```python
from build123d import *

# Parameters (mm, degrees)
F9_DEPTH = 60


with BuildPart() as f3:
    # F0 (on Top) → F3 section 0
    with BuildSketch(Plane.XY):
        Polygon((75, 43.3012701892), (0, 86.6025403784), (-75, 43.3012701892), (-75, -43.3012701892), (0, -86.6025403784), (75, -43.3012701892), align=None)
    # F2 (on offset) → F3 section 1
    with BuildSketch(Plane.XY.offset(50)):
        Polygon((40.3265245185, 23.2825297862), (0, 46.5650595725), (-40.3265245185, 23.2825297862), (-40.3265245185, -23.2825297862), (0, -46.5650595725), (40.3265245185, -23.2825297862), align=None)
    loft()

    # F3_face (on face) → F6 section 0
    with BuildSketch(Plane.XY.offset(50), mode=Mode.PRIVATE) as f6_s0:
        Polygon((40.3265245185, -23.2825297862), (40.3265245185, 23.2825297862), (0, 46.5650595725), (-40.3265245185, 23.2825297862), (-40.3265245185, -23.2825297862), (0, -46.5650595725), align=None)
    loft([f6_s0.sketch, Vertex(-50.6460405886, 55.1455877721, 115)])

    # F8 (on offset) → F9 (join)
    with BuildSketch(Plane(origin=(15.7716130811, -27.3172351738, 55.0342066068), x_dir=(0.9685974066, 0.1105451644, -0.2227079489), z_dir=(0.2486343981, -0.4306474099, 0.8675965332))):
        Polygon((25.1611340791, 2.2766380571), (-68.6507374048, 100.4471331835), (-16.3836460561, -19.314782694), align=None)
    extrude(amount=F9_DEPTH)


solid = f3.part
```
Geometry: final body of the model. Coordinates: model frame, mm. A direction names the side the tool comes from. Coordinates: 2 decimals unless noted, no trailing zeros. Order: outer loops, then holes, each group sorted by start corner. A loop starts at its lowest first (then second) coordinate and runs counter-clockwise, first axis right, second up. Notation, with made-up numbers: (-7, 52) -> (47, 52) arc R25 cw to (47, 84) -> close; hole circle Ø6 at (61, 22). An arc over 180 degrees is marked (long way). Answer in a Markdown table with one row per item.
Item 1: Section B-B on z = 93. Output: boundary loops of the cut face in (x, y), plus the area to 3 significant figures.
Return value:
| item | result |
|---|---|
| outline | (-47.15, 28.6) -> (-33.5, 20.72) -> (-33.57, 20.68) -> (12.2, -67.73) -> (52.34, -43.62) -> (-19.77, 28.65) -> (-19.86, 28.6) -> (-19.86, 44.36) -> (-33.5, 52.24) -> (-47.15, 44.36) -> close |
| area | 3,760 mm² |
Item 2: Section C-C on z = 130. Output: boundary loops of the cut face in (x, y).
Return value:
| item | result |
|---|---|
| outline | (-46.42, 47.61) -> (-6.91, -28.71) -> (16.34, -15.28) -> close |
Item 3: Contact query for flat-ended pins moving along their axis: P1, Ø3, axis at y = -16.5, z = 29, coming from the +X side; P2, Ø1.5, axis at y = -40.5, z = 42, coming from the +X side; P3, Ø5, axis at x = -10.5, y = 2, coming from the +Z side. Output: stop coordinate, or through.
Return value:
| item | result |
|---|---|
| P1 | stops at x = 55.93 |
| P2 | stops at x = 23.26 |
| P3 | stops at z = 147.7 |
Item 4: Section A-A on z = 74.5. Output: boundary loops of the cut face in (x, y).
Return value:
| item | result |
|---|---|
| outline | (-44.22, 6.28) -> (-19.09, -8.23) -> (-19.14, -8.26) -> (6.9, -58.54) -> (47.04, -34.44) -> (6.27, 6.41) -> (6.04, 6.28) -> (6.04, 35.29) -> (-19.09, 49.8) -> (-44.22, 35.29) -> close |
Item 5: Ray query, L1, parallel to X at y = 33, z = 14.5; L2, parallel to Z at x = -63, y = -17; L3, parallel to X at y = 14, z = 141. Return the intervals inside material, ascending.
Return value:
| item | result |
|---|---|
| L1 | x = -64.94 to 64.94 |
| L2 | z = 0 to 17.3 |
| L3 | x = -28.69 to -15.18 |
Item 6: Access query for faces 1 (the flat face through (-43.98, 19.02, 73.02)), 2 (the flat face through (27.095, -47.369, 75.93)), 3 (the flat face through (1, 2, 0)), 4 (the flat face through (-30.845, 43.73, 75.733)). Directions: +Z, -Z, +X, -X, +Y, -Y. A direction counts if a zero-diameter tool reaches every point of the face in a straight line with its end or side. Return the directions, or none.
Return value:
| item | result |
|---|---|
| face 1 | -X, +Y, -Y |
| face 2 | +X, -Y |
| face 3 | -Z, +X, -X, +Y, -Y |
| face 4 | -X, +Y |
